Design review of the part built by this model. Coordinates are the model's own, in mm. Face numbers are marked on the shaded views. A direction names the side the tool comes from. Round coordinates to 2 decimals unless told otherwise and drop trailing zeros. Write each loop counter-clockwise with the first axis right and the second up, starting at its lowest first coordinate (ties: lowest second). Pieces come first, ordered by that corner, then holes. Notation, with made-up numbers: (47.5, 42) -> (97.5, 42) arc R29 cw to (97.5, 74) -> close; hole circle Ø4 at (28, -28). An arc over 180 degrees is marked (long way). One line per question, with ' | ' between items. Start each with the question number.
1) Consider section B-B (y = -2). Give the boundary of the cut face in (x, z), then the cut area to 3 significant figures.
2) Mouldability with a two-part tool opening along Y and no side actions: class the marked faces 1, 2 and 3 as +Y half, -Y half, draft (parallel to the pull), parting line (faces both ways), or undercut.
3) Consider section A-A (x = -0.75). Give the boundary of the cut face in (y, z), then the cut area to 3 significant figures.
4) For probe 1 along Y at (x, z) = (1.98, 0.65); probe 2 along X at (y, z) = (-8.75, 0.6); probe 3 along X at (y, z) = (-9.5, 1.2), list the stretches that pass through material, from the lowest coordinate up.
5) Consider section C-C (z = 1.1). Count the separate pieces of the cut face and the enclosed holes in it, then the cut area to 3 significant figures.
6) For the marked faces 4 and 5, list the 3-axis set-ups (+Z, -Z, +X, -X, +Y, -Y) from which the entire face can be reached by the end or side of a thin tool; tool diameter is ignored.
7) Insertion check: pin 1 Ø0.6 at (y, z) = (-9.5, 0.5) entering from -X. The pin has a flat end and moves straight along its axis. Give the tip position at first contact, or say it passes through.
8) Consider section D-D (x = 8.75). Give the boundary of the cut face in (y, z).
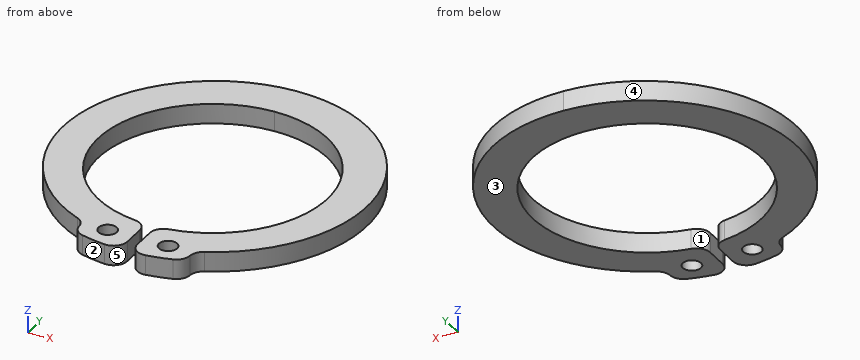
Autodesk Inventor part; units mm, degrees
ref_plane "YZ Plane" through (0, 0, 0) normal (1, 0, 0) x (0, 1, 0)
ref_plane "XZ Plane" through (0, 0, 0) normal (0, 1, 0) x (-1, 0, 0)
ref_plane "XY Plane" through (0, 0, 0) normal (0, 0, 1) x (1, 0, 0)
sketch "Sketch1" plane through (0, 0, 0) normal (0, 0, 1) x (1, 0, 0)
  arc A0 (0, 7.5) -> (-0.33, -7.4927) centre (0, 0) ccw
  line L0 (0, -10.4012) -> (0, 10.52)
  line L1 (-0.33, -7.4927) -> (-0.33, -10.7927)
  arc A1 (-3.63, -10.1693) -> (-0.33, -10.7927) centre (0, 0) ccw
  arc A2 (0, 10.2) -> (-3.63, -8.9927) centre (0, 0.2604) ccw
  line L2 (-3.63, -8.9927) -> (-3.63, -10.1693)
  line L3 (0, 10.2) -> (0, 7.5)
  arc A3 (0.33, -7.4927) -> (0, 7.5) centre (0, 0) ccw
  line L4 (0.33, -7.4927) -> (0.33, -10.7927)
  arc A4 (0.33, -10.7927) -> (3.63, -10.1693) centre (0, 0) ccw
  arc A5 (3.63, -8.9927) -> (0, 10.2) centre (0, 0.2604) ccw
  line L5 (3.63, -8.9927) -> (3.63, -10.1693)
  line L6 (0, 10.2) -> (0, 7.5)
  dimension "d0" = 15
  dimension "d11" = 3.3
  dimension "d21" = 0.33
  dimension "d22" = 3.3
  dimension "d25" = 2.7
  dimension "d26" = 1.5
extrude "Extrusion1" add sketch "Sketch1" along normal blind 1.3
sketch "Sketch3" plane through (0, 0, 1.3) normal (0, 0, 1) x (1, 0, 0)
  line L0 (-0.33, -7.4927) -> (-0.33, -10.7927)
  line L1 (0, -14.9913) -> (0, 14.3985)
  point P0 (-1.98, -9.1427)
  point P1 (1.98, -9.1427)
  dimension "d30" = 1.65
  dimension "d31" = 1.65
hole "Hole1" at (-1.98, -9.1427, 1.3) at (1.98, -9.1427, 1.3) direction (0, 0, -1) diameter 1.2 end through all
fillet "Fillet1" radius 0.9 8 edges at (0.33, -7.4927, 0.65) (-0.33, -7.4927, 0.65) (0.33, -10.7927, 0.65) (3.63, -10.1693, 0.65) (-3.63, -10.1693, 0.65) (-3.63, -8.9927, 0.65) (-0.33, -10.7927, 0.65) (3.63, -8.9927, 0.65)
equation "\"d32\" = Diam5"
equation "\"d39\" = 0.333333 * b"
equation "\"d0\" = Dg"
equation "\"d11\" = ParA"
equation "\"d21\" = 0.1 * ParA"
equation "\"d22\" = ParA"
equation "\"d25\" = b"
equation "\"d26\" = ParJ"
equation "\"d27\" = tt"
equation "\"b\" = 2.7"
equation "\"Dg\" = 15"
equation "\"ParJ\" = 1.5"
equation "\"ParA\" = 3.3"
equation "\"tt\" = 1.3"
equation "\"Diam5\" = 1.2"
equation "\"TEMPLATE\" = 1.2345"
properties part number "ANSI B27.8M - 3DM1-3DM1-16" material "Steel, Mild"
From the geometry:
1) outline: (-9.68, 0) -> (-7.23, 0) -> (-7.23, 1.3) -> (-9.68, 1.3) -> close; (7.23, 0) -> (9.68, 0) -> (9.68, 1.3) -> (7.23, 1.3) -> close | area: 6.37 mm2
2) face 1: undercut | face 2: -Y half | face 3: draft
3) outline: (-10.58, 0) -> (-7.55, 0) -> (-7.55, 1.3) -> (-10.58, 1.3) -> close; (7.46, 0) -> (10.17, 0) -> (10.17, 1.3) -> (7.46, 1.3) -> close | area: 7.47 mm2
4) probe 1: y = -10.61 to -9.74, -8.54 to -7.23, 7.23 to 10 | probe 2: x = -4.2 to -2.43, -1.53 to -0.33, 0.33 to 1.53, 2.43 to 4.2 | probe 3: x = -3.63 to -2.46, -1.5 to -0.33, 0.33 to 1.5, 2.46 to 3.63
5) separate pieces: 1 | enclosed holes: 2 | area: 137 mm2
6) face 4: +Z, -Z, -X | face 5: +Z, -Z, -Y
7) pin 1: stops at x = -3.72
8) outline: (-4.45, 0) -> (4.98, 0) -> (4.98, 1.3) -> (-4.45, 1.3) -> close
